For this review, take the finished solid that the model builds, in its own axes (mm). A direction names the side the tool comes from. Coordinates: 2 decimals unless noted, no trailing zeros. Loops run counter-clockwise (first coordinate to the right, second up) from the corner with the lowest first, then second, coordinate; pieces in that order, holes last. Notation, with made-up numbers: M -35,56 L 6,56 A24 cw 6,85 Z; hole C 80.5,17.25 d2. An arc over 180 degrees is marked long. Put each result on its own line as item: value.
```python
from build123d import *

# Parameters (mm, degrees)
SKETCH1_W           = 304.8
SKETCH1_H           = 381
BOSS_EXTRUDE1_DEPTH = 6.35
SKETCH2_W           = 6.35
SKETCH2_H           = 25.019
SKETCH2_W_2         = 25.019
SKETCH2_H_2         = 6.35
CUT_EXTRUDE3_DEPTH  = 6.35


with BuildPart() as part:
    # Sketch1 → Boss-Extrude1 (new body)
    with BuildSketch(Plane.XY):
        with Locations((152.4, -190.5)):
            Rectangle(SKETCH1_W, SKETCH1_H)
    extrude(amount=BOSS_EXTRUDE1_DEPTH)

    # Sketch2 → Cut-Extrude3 (cut)
    with BuildSketch(Plane.XY):
        with Locations((301.625, -38.1)):
            Rectangle(SKETCH2_W, SKETCH2_H)
        with BuildLine():
            Line((240.70945, -50.8), (240.70945, -355.600000025))
            ThreePointArc((240.70945, -355.600000025), (251.720356878, -366.610893146), (262.73125, -355.599986268))
            Line((262.73125, -355.599986268), (262.73125, -50.8))
            ThreePointArc((262.73125, -50.8), (251.72035, -39.7891), (240.70945, -50.8))
        make_face()
        with Locations((3.175, -38.1)):
            Rectangle(SKETCH2_W, SKETCH2_H)
        with Locations((301.625, -88.9)):
            Rectangle(SKETCH2_W, SKETCH2_H)
        with Locations((301.625, -139.7)):
            Rectangle(SKETCH2_W, SKETCH2_H)
        with Locations((301.625, -190.5)):
            Rectangle(SKETCH2_W, SKETCH2_H)
        with Locations((301.625, -241.3)):
            Rectangle(SKETCH2_W, SKETCH2_H)
        with Locations((301.625, -292.1)):
            Rectangle(SKETCH2_W, SKETCH2_H)
        with Locations((301.625, -342.9)):
            Rectangle(SKETCH2_W, SKETCH2_H)
        with Locations((3.175, -88.9)):
            Rectangle(SKETCH2_W, SKETCH2_H)
        with Locations((3.175, -139.7)):
            Rectangle(SKETCH2_W, SKETCH2_H)
        with Locations((3.175, -190.5)):
            Rectangle(SKETCH2_W, SKETCH2_H)
        with Locations((3.175, -241.3)):
            Rectangle(SKETCH2_W, SKETCH2_H)
        with Locations((3.175, -292.1)):
            Rectangle(SKETCH2_W, SKETCH2_H)
        with Locations((3.175, -342.9)):
            Rectangle(SKETCH2_W, SKETCH2_H)
        with Locations((101.6, -377.825)):
            Rectangle(SKETCH2_W_2, SKETCH2_H_2)
        with Locations((50.8, -377.825)):
            Rectangle(SKETCH2_W_2, SKETCH2_H_2)
        with Locations((152.4, -377.825)):
            Rectangle(SKETCH2_W_2, SKETCH2_H_2)
        with Locations((203.2, -377.825)):
            Rectangle(SKETCH2_W_2, SKETCH2_H_2)
        with Locations((254, -377.825)):
            Rectangle(SKETCH2_W_2, SKETCH2_H_2)
        with BuildLine():
            Line((42.136581375, -50.947063112), (42.542981176, -355.746778447))
            ThreePointArc((42.542981176, -355.746778447), (53.568545713, -366.742994354), (64.56476162, -355.717429817))
            Line((64.56476162, -355.717429817), (64.1583618, -50.917700725))
            ThreePointArc((64.1583618, -50.917700725), (53.132790394, -39.921491706), (42.136581375, -50.947063112))
        make_face()
    extrude(amount=CUT_EXTRUDE3_DEPTH, mode=Mode.SUBTRACT)


solid = part.part
```
(1) Draft analysis for pull direction Y (two halves, no side actions). For faces 1 (the cylindrical face through (53.375, -39.924, 3.131)), 2 (the flat face through (150, -188, 6.35)), 3 (the cylindrical face through (251.96, -39.79, 3.13)), state which applies: +Y half, -Y half, draft (parallel to the pull), parting line (faces both ways), or undercut.
Determined:
face 1: undercut
face 2: draft
face 3: undercut
(2) Add section C-C (x = 203.5). Write out the cut boundary in (y, z).
Determined:
outline: M -374.65,0 L 0,0 L 0,6.35 L -374.65,6.35 Z
(3) For pin 1 (3 mm diameter, centred on y = -134.5, z = 5, fed in from -X), flat-tipped, find the tip position at first contact; note if it passes through.
Determined:
pin 1: stops at x = 6.35
(4) Tool access review of faces 4 (the cylindrical face through (53.33, -366.74, 3.13)), 5 (the flat face through (150, -188, 0)): name each direction out of +Z, -Z, +X, -X, +Y, -Y from which nothing blocks a thin tool from reaching the whole face with its end or side.
Determined:
face 4: +Z, -Z
face 5: -Z, +X, -X, +Y, -Y
(5) Add section B-B (z = 4.5). State how many separate pieces and enclosed holes the cut face has, plus the area to 3 significant figures.
Determined:
separate pieces: 1
enclosed holes: 2
area: 98,900 mm^2
(6) Add section A-A (y = -72). Write out the cut boundary in (x, z).
Determined:
outline: M 0,0 L 42.16,0 L 42.16,6.35 L 0,6.35 Z; M 64.19,0 L 240.71,0 L 240.71,6.35 L 64.19,6.35 Z; M 262.73,0 L 304.8,0 L 304.8,6.35 L 262.73,6.35 Z
(7) Wall thickness on line 1 along X through (y, z) = (-84, 3); line 2 along X through (y, z) = (-316, 3.5); line 3 along Y through (x, z) = (145.5, 2.25): over which ranges is each line inside the solid? List them lowest first. Write a range as [from, to].
Determined:
line 1: x = [6.35, 42.18], [64.2, 240.71], [262.73, 298.45]
line 2: x = [0, 42.49], [64.51, 240.71], [262.73, 304.8]
line 3: y = [-374.65, 0]
